Build history of the part. All positions in model axes, mm. A direction names the side the tool comes from. Give positions to 0.01 mm unless a question says otherwise; leave off trailing zeros. Loops run counter-clockwise (first coordinate to the right, second up) from the corner with the lowest first, then second, coordinate; pieces in that order, holes last. Notation, with made-up numbers: (10, -6) -> (54, -6) arc R21 cw to (54, 1) -> close; hole circle Ø4 at (16, 40.5). An arc over 180 degrees is marked (long way). Answer as a JSON object with one key per item and string values. Group by question number.
Q1. Tool access for faces 4 (the cylindrical face through (-14.88, 65.22, -47.24)), 5 (the conical face through (-5.97, 142.83, -18.97)), 6 (the cylindrical face through (5.796, 165.709, 7.559)): list every direction of +Z, -Z, +X, -X, +Y, -Y with a clear straight run to the whole face (end or side of a thin tool).
Q2. Band-saw the part on A-A, the plane y = 47.5. Write the cut outline in (x, z).
Q3. Two-plate mould, pull along Z, no slides. Class faces 1 (the conical face through (7.024, -22.685, 9.161)), 2 (the flat face through (7, 171.45, -7)), 3 (the cylindrical face through (-29.18, 65.22, 31.83)): pulls with the +Z half, pulls with the -Z half, needs draft (parallel to the pull), parting line crosses it, or undercut.
Q4. Drop flat-ended pins along their axis: pin 1 (1.5 mm diameter, centred on x = 31.5, y = 111.5, fed in from -Z); pin 2 (12 mm diameter, centred on x = 8, y = 67, fed in from +Z); pin 3 (4 mm diameter, centred on x = 12.5, y = 8, fed in from +Z). Give the stop position or say it passes through.
Q5. Wall check: probe 1 along X at (y, z) = (167.5, 0) (3 decimals); probe 2 along Z at (x, y) = (-1, 69.5); probe 3 along Y at (x, z) = (26, 12) (3 decimals). Give the ranges that are in metal, low to high. Write a range as from..to.
from build123d import *

# Parameters (mm, degrees)
SHELL1_T = -6.35


with BuildPart() as part:
    # Sketch1 → Revolve1 (revolve)
    with BuildSketch(Plane.XY, mode=Mode.PRIVATE) as revolve1_sk:
        with BuildLine():
            Line((-10.034098989, -23.334027888), (-34.164098989, -12.957644961))
            ThreePointArc((-34.164098989, -12.957644961), (-45.343511193, -3.593117524), (-49.53, 10.376382927))
            Line((-49.53, 10.376382927), (-49.53, 118.540573173))
            ThreePointArc((-49.53, 118.540573173), (-46.072705707, 131.334230439), (-36.641994784, 140.645097292))
            Line((-36.641994784, 140.645097292), (-22.319002608, 148.752451354))
            ThreePointArc((-22.319002608, 148.752451354), (-17.603647146, 153.40788478), (-15.875, 159.804713413))
            Line((-15.875, 159.804713413), (-15.875, 171.45))
            Line((-15.875, 171.45), (0, 171.45))
            Line((0, 171.45), (0, -25.4))
            ThreePointArc((0, -25.4), (-5.122289119, -24.878146116), (-10.034098989, -23.334027888))
        make_face()
    revolve(revolve1_sk.sketch.rotate(Axis((0, 0, 0), (0, 1, 0)), 270), axis=Axis((0, 0, 0), (0, 1, 0)))

    # Shell1
    shell1_openings = [part.faces().sort_by_distance(p)[0] for p in [
        (0, 171.45, 0),
    ]]
    offset(amount=SHELL1_T, openings=shell1_openings, kind=Kind.INTERSECTION)


solid = part.part
Worked answers:
{
 "1": {"face 4": "+Y, -Y", "face 5": "none", "face 6": "+Y"},
 "2": {"outline": "circle Ø99.06 at (0, 0); hole circle Ø86.36 at (0, 0)"},
 "3": {"face 1": "parting line crosses it", "face 2": "needs draft", "face 3": "undercut"},
 "4": {"pin 1": "z = -38.83", "pin 2": "z = 49.49", "pin 3": "z = 48.32"},
 "5": {"probe 1": "-15.875..-9.525, 9.525..15.875", "probe 2": "-49.52..-43.17, 43.17..49.52", "probe 3": "-15.335..-8.423, 137.88..145.177"}
}
